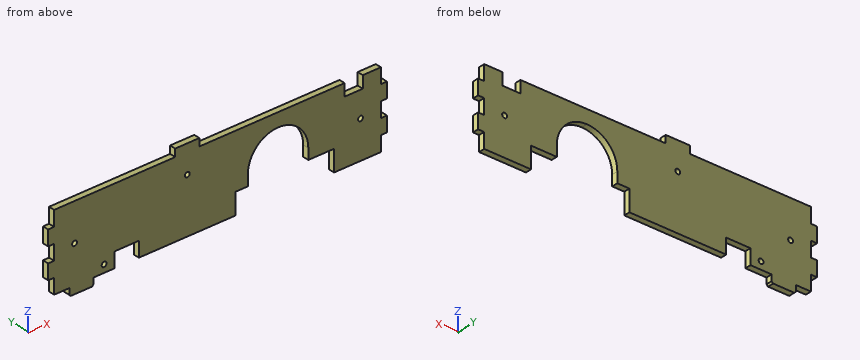
Autodesk Fusion 360 part; units mm, degrees
sketch "スケッチ1" plane through (0, 0, 0) normal (0, 1, 0) x (1, 0, 0)
  line L0 (-20, -14) -> (-20, -41)
  line L1 (-20, -41) -> (20, -41)
  line L2 (20, -41) -> (20, -14)
  line L3 (20, -14) -> (37, -14)
  line L4 (37, -14) -> (37, 0)
  line L5 (37, 0) -> (68, 0)
  line L6 (68, 0) -> (68, -10)
  line L7 (68, -10) -> (72, -10)
  line L8 (72, -10) -> (72, -20)
  line L9 (72, -20) -> (68, -20)
  line L10 (68, -20) -> (68, -30)
  line L11 (68, -30) -> (72, -30)
  line L12 (72, -30) -> (72, -40)
  line L13 (72, -40) -> (68, -40)
  line L14 (68, -40) -> (68, -50)
  line L15 (68, -50) -> (-148, -50)
  line L16 (-148, 0) -> (-28, 0)
  line L17 (-148, 0) -> (-148, -10)
  line L18 (-148, -10) -> (-152, -10)
  line L19 (-152, -10) -> (-152, -20)
  line L20 (-152, -20) -> (-148, -20)
  line L21 (-148, -20) -> (-148, -30)
  line L22 (-148, -30) -> (-152, -30)
  line L23 (-152, -30) -> (-152, -40)
  line L24 (-152, -40) -> (-148, -40)
  line L25 (-148, -40) -> (-148, -50)
  line L26 (-108, 0) -> (-92, 0)
  line L27 (-92, 0) -> (-92, -10)
  line L28 (-92, -10) -> (-108, -10)
  line L29 (-108, -10) -> (-108, 0)
  line L30 (-68, -50) -> (-52, -50)
  line L31 (-52, -50) -> (-52, -55)
  line L32 (-52, -55) -> (-68, -55)
  line L33 (-68, -55) -> (-68, -50)
  line L34 (-138, 0) -> (-122, 0)
  line L35 (-122, 0) -> (-122, 5)
  line L36 (-122, 5) -> (-138, 5)
  line L37 (-138, 5) -> (-138, 0)
  line L38 (56, -50) -> (44, -50)
  line L39 (44, -50) -> (44, -42)
  line L40 (44, -42) -> (56, -42)
  line L41 (56, -42) -> (56, -50)
  line L42 (-28, 0) -> (-28, -14)
  line L43 (-28, -14) -> (-20, -14)
  point P0 (-100, 0)
  point P1 (-130, 0)
  point P2 (-60, -50)
  dimension "d9" = 20
  dimension "d10" = 14
  dimension "d11" = 68
  dimension "d12" = 4
  dimension "d13" = 10
  dimension "d14" = 10
  dimension "d15" = 10
  dimension "d16" = 10
  dimension "d17" = 10
  dimension "d19" = 17
  dimension "d34" = 4
  dimension "d37" = 216
  dimension "d40" = 100
  dimension "d41" = 10
  dimension "d42" = 16
  dimension "d43" = 5
  dimension "d44" = 16
  dimension "d45" = 60
  dimension "d46" = 130
  dimension "d50" = 12
  dimension "d51" = 12
  dimension "d52" = 8
  dimension "d53" = 41
  dimension "d54" = 20
  dimension "d55" = 8
extrude "押し出し1" add sketch "スケッチ1" along normal blind 4 contours L0 L1 L2 L3 L4 L5 L6 L7 L8 L9 L10 L11 L12 L13 L14 L15 L16 L17 L18 L19 L20 L21 L22 L23 L24 L25 L27 L28 L29 L30 L34 L39 L40 L41 L42 L43 | L16 L34 L35 L36 L37 | L15 L30 L31 L32 L33
sketch "スケッチ2" plane through (0, 4, 0) normal (0, 1, 0) x (-1, 0, 0)
  line L0 (-56, 50) -> (-68, 50)
  line L1 (-68, 50) -> (-68, 40)
  line L2 (-68, 40) -> (-72, 40)
  line L3 (-72, 40) -> (-72, 30)
  line L4 (-72, 30) -> (-68, 30)
  line L5 (-68, 30) -> (-68, 20)
  line L6 (-68, 20) -> (-72, 20)
  line L7 (-72, 20) -> (-72, 10)
  line L8 (-72, 10) -> (-68, 10)
  line L9 (-68, 10) -> (-68, 0)
  line L10 (-68, 0) -> (-37, 0)
  line L11 (-37, 0) -> (-37, 14)
  line L12 (-37, 14) -> (-20, 14)
  line L13 (-20, 14) -> (-20, 41)
  line L14 (-20, 41) -> (20, 41)
  line L15 (20, 41) -> (20, 14)
  line L16 (138, 0) -> (148, 0)
  line L17 (-54.5, 25) -> (-68, 25)
  line L18 (60, 36.5) -> (115, 5)
  line L19 (148, 0) -> (148, 10)
  line L20 (148, 10) -> (152, 10)
  line L21 (152, 10) -> (152, 20)
  line L22 (152, 20) -> (148, 20)
  line L23 (148, 20) -> (148, 30)
  line L24 (148, 30) -> (152, 30)
  line L25 (152, 30) -> (152, 40)
  line L26 (152, 40) -> (148, 40)
  line L27 (148, 40) -> (148, 50)
  line L28 (148, 25) -> (134.5, 25)
  line L29 (92, 0) -> (92, 10)
  line L30 (92, 10) -> (108, 10)
  line L31 (108, 10) -> (108, 0)
  line L32 (122, 0) -> (122, -5)
  line L33 (122, -5) -> (138, -5)
  line L34 (138, -5) -> (138, 0)
  line L35 (68, 50) -> (68, 55)
  line L36 (68, 55) -> (52, 55)
  line L37 (52, 55) -> (52, 50)
  line L38 (52, 50) -> (-44, 50)
  line L39 (108, 0) -> (122, 0)
  line L40 (-44, 50) -> (-44, 42)
  line L41 (-44, 42) -> (-56, 42)
  line L42 (-56, 42) -> (-56, 50)
  line L43 (148, 50) -> (68, 50)
  line L44 (20, 14) -> (28, 14)
  line L45 (28, 14) -> (28, 0)
  line L46 (28, 0) -> (92, 0)
  dimension "d24" = 13.5
  dimension "d25" = 5
  dimension "d27" = 13.5
  dimension "d38" = 60
  dimension "d39" = 115
hole "穴1" at (-115, 4, 5) at (-60, 4, 36.5) at (54.5, 4, 25) at (-134.5, 4, 25) direction (0, -1, 0) diameter 3.2 end through all
fillet "フィレット1" radius 20 2 edges at (20, 2, 41) (-20, 2, 41)
chamfer "面取り1" distance 1 angle 45 2 edges at (-138, 2, -5) (-122, 2, -5)
Could you check a few things on this model? Use its own coordinates, in mm. Give positions to 0.01 mm unless a question says otherwise; leave off trailing zeros. Answer as CSV lines item,"result". Start each with the question number.
(1) I need wall thicknesses on probe 1 along X at (y, z) = (1.4, 5); probe 2 along X at (y, z) = (0.45, 1); probe 3 along Z at (x, y) = (-134.5, 2.1). Which ranges of each line are inside material? Lowest first, please.
(2) I'm going to push flat-ended pins straight in: pin 1 Ø1 at (x, y) = (-105.5, 0.5) entering from +Z; pin 2 Ø1.2 at (x, y) = (69, 2) entering from +Z; pin 3 Ø2 at (x, y) = (-149.5, 3) entering from -Z. Where does each tip first touch, or does it pass through?
(3) If we section it at A-A on y = 1.75: Count the separate pieces of the cut face and the enclosed holes in it, then the cut area to 3 significant figures.
Computed:
1,probe 1,"x = -148 to -116.6, -113.4 to -108, -92 to -28, 37 to 68"
1,probe 2,"x = -148 to -108, -92 to -28, 37 to 68"
1,probe 3,"z = -5 to 23.4, 26.6 to 50"
2,pin 1,"stops at z = 50"
2,pin 2,"stops at z = 40"
2,pin 3,"stops at z = 10"
3,separate pieces,"1"
3,enclosed holes,"4"
3,area,"9,010 mm2"
